Autodesk Fusion 360 part; units mm, degrees
sketch "Sketch1" plane through (0, 0, 0) normal (0, 0, 1) x (1, 0, 0)
  line L0 (-5.5, -3.1754) -> (0, -6.3509)
  line L1 (0, -6.3509) -> (5.5, -3.1754)
  line L2 (5.5, -3.1754) -> (5.5, 3.1754)
  line L3 (5.5, 3.1754) -> (0, 6.3509)
  line L4 (0, 6.3509) -> (-5.5, 3.1754)
  line L5 (-5.5, 3.1754) -> (-5.5, -3.1754)
  dimension "d1" = 5.5
extrude "Extrude1" add sketch "Sketch1" along normal blind 5
sketch "Sketch2" plane through (0, 0, 5) normal (0, 0, 1) x (-1, 0, 0)
  line L0 (5.5, -3.1754) -> (5.5, 3.1754)
  line L1 (5.5, 3.1754) -> (0, 6.3509)
  line L2 (0, 6.3509) -> (-5.5, 3.1754)
  line L3 (-5.5, 3.1754) -> (-5.5, -3.1754)
  line L4 (-5.5, -3.1754) -> (0, -6.3509)
  line L5 (0, -6.3509) -> (5.5, -3.1754)
  circle A0 centre (0, 0) radius 2
  dimension "d4" = 4
extrude "Extrude2" cut sketch "Sketch2" against normal blind 12 contours A0
extrude "Extrude3" add 1 faces at (-4.3333, 0, 5) along direction (0, 0, 1) blind 25
sketch "Sketch3" plane through (0, 0, 30) normal (0, 0, 1) x (-1, 0, 0)
  circle A0 centre (0, 0) radius 2
  line L0 (5.5, -3.1754) -> (5.5, 3.1754)
  line L1 (5.5, 3.1754) -> (0, 6.3509)
  line L2 (0, 6.3509) -> (-5.5, 3.1754)
  line L3 (-5.5, 3.1754) -> (-5.5, -3.1754)
  line L4 (-5.5, -3.1754) -> (0, -6.3509)
  line L5 (0, -6.3509) -> (5.5, -3.1754)
  line L6 (-5.8, -3.3486) -> (0, -6.6973)
  line L7 (0, -6.6973) -> (5.8, -3.3486)
  line L8 (5.8, -3.3486) -> (5.8, 3.3486)
  line L9 (5.8, 3.3486) -> (0, 6.6973)
  line L10 (0, 6.6973) -> (-5.8, 3.3486)
  line L11 (-5.8, 3.3486) -> (-5.8, -3.3486)
  dimension "d9" = 5.8
extrude "Extrude4" add sketch "Sketch3" against normal blind 16 contours L6 L7 L8 L9 L10 L11
sketch "Sketch4" plane through (0, 0, 30) normal (0, 0, 1) x (-1, 0, 0)
  line L0 (-5.8, 3.3486) -> (-5.8, -3.3486)
  line L1 (-5.8, -3.3486) -> (0, -6.6973)
  line L2 (0, -6.6973) -> (5.8, -3.3486)
  line L3 (5.8, -3.3486) -> (5.8, 3.3486)
  line L4 (5.8, 3.3486) -> (0, 6.6973)
  line L5 (0, 6.6973) -> (-5.8, 3.3486)
  circle A0 centre (0, 0) radius 2
  circle A1 centre (0, 0) radius 2.65
  dimension "d12" = 5.3
extrude "Extrude5" cut sketch "Sketch4" against normal blind 35 contours A1
extrude "Extrude6" cut 1 faces at (-2.275, -3.9404, 0) along direction (0, 0, 1) blind 2
extrude "Extrude7" cut 1 faces at (2.375, -4.1136, 30) along direction (0, 0, -1) blind 33 from surface at 12
sketch "Sketch5" plane through (0, 0, 30) normal (0, 0, 1) x (-1, 0, 0)
  circle A0 centre (0, 0) radius 2.65
  line L0 (-5.8, 3.3486) -> (-5.8, -3.3486)
  line L1 (-5.8, -3.3486) -> (0, -6.6973)
  line L2 (0, -6.6973) -> (5.8, -3.3486)
  line L3 (5.8, -3.3486) -> (5.8, 3.3486)
  line L4 (5.8, 3.3486) -> (0, 6.6973)
  line L5 (0, 6.6973) -> (-5.8, 3.3486)
  line L6 (-6.1, -3.5218) -> (0, -7.0437)
  line L7 (0, -7.0437) -> (6.1, -3.5218)
  line L8 (6.1, -3.5218) -> (6.1, 3.5218)
  line L9 (6.1, 3.5218) -> (0, 7.0437)
  line L10 (0, 7.0437) -> (-6.1, 3.5218)
  line L11 (-6.1, 3.5218) -> (-6.1, -3.5218)
  dimension "d20" = 6.1
extrude "Extrude8" add sketch "Sketch5" against normal blind 12 contours L6 L7 L8 L9 L10 L11
sketch "Sketch6" plane through (0, 0, 30) normal (0, 0, 1) x (-1, 0, 0)
  line L0 (-6.1, 3.5218) -> (-6.1, -3.5218)
  line L1 (-6.1, -3.5218) -> (0, -7.0437)
  line L2 (0, -7.0437) -> (6.1, -3.5218)
  line L3 (6.1, -3.5218) -> (6.1, 3.5218)
  line L4 (6.1, 3.5218) -> (0, 7.0437)
  line L5 (0, 7.0437) -> (-6.1, 3.5218)
  circle A0 centre (0, 0) radius 2.65
  line L6 (-6, -3.4641) -> (0, -6.9282)
  line L7 (0, -6.9282) -> (6, -3.4641)
  line L8 (6, -3.4641) -> (6, 3.4641)
  line L9 (6, 3.4641) -> (0, 6.9282)
  line L10 (0, 6.9282) -> (-6, 3.4641)
  line L11 (-6, 3.4641) -> (-6, -3.4641)
  circle A1 centre (0, 0) radius 2.85
  dimension "d23" = 6
  dimension "d24" = 5.7
extrude "Extrude9" cut sketch "Sketch6" against normal blind 13
For this review, take the finished solid that the model builds, in its own axes (mm). Give positions to 0.01 mm unless a question says otherwise; leave off trailing zeros. Write each loop counter-clockwise with the first axis right and the second up, starting at its lowest first coordinate (ties: lowest second). Pieces come first, ordered by that corner, then holes. Notation, with made-up numbers: (64, 25) -> (102, 25) arc R31 ccw to (102, 49) -> close; hole circle Ø5 at (12.25, 50.5). An arc over 180 degrees is marked (long way). Use CSV: the item, a comma, the result in double quotes.
Q1. Take a section at D-D, the plane y = -3.75. Write out the cut boundary in (x, z), then the cut area to 3 significant figures.
Conclusion:
outline,"(-5.5, 18) -> (5.5, 18) -> (5.5, 30) -> (-5.5, 30) -> close"
area,"132 mm2"
Q2. Take a section at A-A, the plane y = 0. Write out the cut boundary in (x, z).
Conclusion:
outline,"(-6, 18) -> (-2.85, 18) -> (-2.85, 30) -> (-6, 30) -> close; (2.85, 18) -> (6, 18) -> (6, 30) -> (2.85, 30) -> close"
Q3. Mouldability with a two-part tool opening along Y and no side actions: class faces 1 (the face through (-3.042, -5.172, 24.084)), 2 (the face through (2.262, 1.734, 24.084)), 3 (the face through (-6, 0, 24)), 4 (the face through (3.042, 5.172, 24.084)) as pulls with the +Y half, pulls with the -Y half, needs draft (parallel to the pull), parting line crosses it, or undercut.
Conclusion:
face 1,"pulls with the -Y half"
face 2,"undercut"
face 3,"needs draft"
face 4,"pulls with the +Y half"
Q4. To check wall thickness, follow probe 1 along X at (y, z) = (0, 23.75); probe 2 along Y at (x, z) = (-1.5, 22); probe 3 along X at (y, z) = (-2.5, 26.5). State the ranges of each line that lie inside material, in increasing order. Write a range as [from, to].
Conclusion:
probe 1,"[-6, -2.85], [2.85, 6]"
probe 2,"[-6.06, -2.42], [2.42, 6.06]"
probe 3,"[-6, -1.37], [1.37, 6]"
Q5. For P1, Ø5, axis at x = 3, z = 26.5, coming from the +Y side; P2, Ø1.5, axis at y = 5, z = 21, coming from the -X side, all flat-tipped, find the tip position at first contact; note any pin that passes through.
Conclusion:
P1,"y = 6.64"
P2,"x = -4.64"
Q6. Take a section at C-C, the plane z = 26. Write out the cut boundary in (x, y), then the cut area to 3 significant figures.
Conclusion:
outline,"(-6, -3.46) -> (0, -6.93) -> (6, -3.46) -> (6, 3.46) -> (0, 6.93) -> (-6, 3.46) -> close; hole circle Ø5.7 at (0, 0)"
area,"99.2 mm2"
Q7. Take a section at B-B, the plane x = 2.5. Write out the cut boundary in (y, z), then the cut area to 3 significant figures.
Conclusion:
outline,"(-5.48, 18) -> (-1.37, 18) -> (-1.37, 30) -> (-5.48, 30) -> close; (1.37, 18) -> (5.48, 18) -> (5.48, 30) -> (1.37, 30) -> close"
area,"98.8 mm2"
